Part model, mm, in its own coordinate system. Coordinates: 2 decimals unless noted, no trailing zeros. Loops run counter-clockwise (first coordinate to the right, second up) from the corner with the lowest first, then second, coordinate; pieces in that order, holes last.
Autodesk Inventor part; units mm, degrees
ref_plane "YZ Plane" through (0, 0, 0) normal (1, 0, 0) x (0, 1, 0)
ref_plane "XZ Plane" through (0, 0, 0) normal (0, 1, 0) x (-1, 0, 0)
ref_plane "XY Plane" through (0, 0, 0) normal (0, 0, 1) x (1, 0, 0)
sketch "スケッチ1" plane through (0, 0, 0) normal (0, 0, 1) x (1, 0, 0)
  circle A0 centre (0, 0) radius 35
  circle A1 centre (0, 0) radius 13.05
  circle A2 centre (0, 0) radius 25 construction
  line L0 (0, 35) -> (0, 0) construction
  line L1 (0, 0) -> (35, 0) construction
  circle A3 centre (25, 0) radius 2.5
  circle A4 centre (0, 25) radius 2.5
  circle A5 centre (-25, 0) radius 2.5
  circle A6 centre (0, -25) radius 2.5
  dimension "d3" = 50
  dimension "d0" = 26.1
  dimension "d1" = 70
  dimension "d2" = 5
  dimension "d6" = 360
extrude "押し出し1" add sketch "スケッチ1" along normal blind 5
properties part number "車軸受け板3"
Q1. Probe line 1 (X direction, y = -1, z = 1.45); line 2 (X direction, y = -25.5, z = 4.3); line 3 (Y direction, x = -8, z = 1.4). List the from-to ranges inside material, lowest first.
Q2. Mould opens along Y. For faces 1 (the cylindrical face through (-0.33, 22.52, 2.46)), 2 (the flat face through (0, -15, 0)), 3 (the cylindrical face through (-28, 21, 2)) say: released by +Y, released by -Y, zero draft, split by the parting line, or undercut.
Q3. Saw through at A-A (y = 0). List the corners of the cut face in (x, z), plus the area to 4 significant figures.
Q4. Drop flat-ended pins along their axis: P1, Ø3, axis at x = 25, y = 0, coming from the +Z side; P2, Ø1, axis at x = 24, z = 4, coming from the +Y side; P3, Ø3, axis at x = 6, z = 2, coming from the -Y side; P4, Ø3, axis at x = 1.5, z = 2, coming from the -Y side. Give the stop position or say it passes through.
Q5. Saw through at D-D (x = -25). List the corners of the cut face in (y, z).
Q6. Saw through at C-C (z = 3.85). List the corners of the cut face in (x, y).
Checked values:
1. line 1: x = -34.99 to -27.29, -22.71 to -13.01, 13.01 to 22.71, 27.29 to 34.99
1. line 2: x = -23.97 to -2.45, 2.45 to 23.97
1. line 3: y = -34.07 to -10.31, 10.31 to 34.07
2. face 1: undercut
2. face 2: zero draft
2. face 3: split by the parting line
3. outline: (-35, 0) - (-27.5, 0) - (-27.5, 5) - (-35, 5) - close; (-22.5, 0) - (-13.05, 0) - (-13.05, 5) - (-22.5, 5) - close; (13.05, 0) - (22.5, 0) - (22.5, 5) - (13.05, 5) - close; (27.5, 0) - (35, 0) - (35, 5) - (27.5, 5) - close
3. area: 169.5 mm2
4. P1: passes through
4. P2: stops at y = 25.94
4. P3: stops at y = -34.71
4. P4: stops at y = -35
5. outline: (-24.49, 0) - (-2.5, 0) - (-2.5, 5) - (-24.49, 5) - close; (2.5, 0) - (24.49, 0) - (24.49, 5) - (2.5, 5) - close
6. outline: circle Ø70 at (0, 0); hole circle Ø5 at (-25, 0); hole circle Ø26.1 at (0, 0); hole circle Ø5 at (0, -25); hole circle Ø5 at (0, 25); hole circle Ø5 at (25, 0)
